Can you work these out from the model? Positions are in its coordinate system, mm. Give positions to 0.01 mm unless a question says otherwise; leave off trailing zeros. Write each loop counter-clockwise with the first axis right and the second up, starting at its lowest first coordinate (ties: lowest second). Pieces come first, ordered by that corner, then holes.
1. If I drill on probe 1 along Z at (x, y) = (89, 5); probe 2 along Z at (x, y) = (81.5, 1.5); probe 3 along X at (y, z) = (4.5, -451), over which ranges is the centre line in solid material (lowest first)?
2. Suppose I cut it at C-C (y = 4.5). Please give me the cut outline in (x, z).
3. I'm going to push flat-ended pins straight in: pin 1 (3 mm diameter, centred on x = 6.5, y = 4.5, fed in from -Z); pin 2 (3 mm diameter, centred on y = 4.5, z = -5, fed in from +X); pin 3 (2 mm diameter, centred on y = 1, z = -626, fed in from -X); pin 4 (3 mm diameter, centred on y = 4, z = -5, fed in from -X). Where does each tip first touch, or does it pass through?
4. Suppose I cut it at B-B (x = 66). Please give me the cut outline in (y, z).
5. Suppose I cut it at A-A (z = -383). Please give me the cut outline in (x, y), and give its area (3 significant figures).
```python
from build123d import *

# Parameters (mm, degrees)
SKETCH1_W           = 219.202
SKETCH1_H           = 879.7036
BOSS_EXTRUDE1_DEPTH = 6.35
SKETCH4_R           = 76.2
SKETCH4_W           = 8.89
SKETCH4_H           = 8.89
CUT_EXTRUDE3_DEPTH  = 907.624653954
FILLET1_R           = 0.254


with BuildPart() as part:
    # Sketch1 → Boss-Extrude1 (new body)
    with BuildSketch(Plane(origin=(0, 0, 0), x_dir=(1, 0, 0), z_dir=(0, 1, 0))):
        with Locations((109.601, 439.8518)):
            Rectangle(SKETCH1_W, SKETCH1_H)
    extrude(amount=BOSS_EXTRUDE1_DEPTH)

    # Sketch4 → Cut-Extrude3 (cut, through all)
    with BuildSketch(Plane(origin=(0, 6.35, 0), x_dir=(1, 0, 0), z_dir=(0, 1, 0))):
        with Locations(Location((86.6394, 439.8518, 0), (0, 0, 270))):
            Circle(SKETCH4_R)
        with Locations((4.445, 4.445)):
            Rectangle(SKETCH4_W, SKETCH4_H)
        with Locations((214.757, 4.445)):
            Rectangle(SKETCH4_W, SKETCH4_H)
        with Locations((214.757, 875.2586)):
            Rectangle(SKETCH4_W, SKETCH4_H)
        with Locations((4.445, 875.2586)):
            Rectangle(SKETCH4_W, SKETCH4_H)
    extrude(amount=-CUT_EXTRUDE3_DEPTH, mode=Mode.SUBTRACT)

    # Fillet1
    fillet1_edges = [part.edges().sort_by_distance(p)[0] for p in [
        (0, 3.175, -870.8136),
        (8.89, 3.175, -879.7036),
        (8.89, 3.175, -870.8136),
        (219.202, 3.175, -870.8136),
        (210.312, 3.175, -870.8136),
        (210.312, 3.175, -879.7036),
        (219.202, 3.175, -8.89),
        (210.312, 3.175, 0),
        (210.312, 3.175, -8.89),
        (0, 3.175, -8.89),
        (8.89, 3.175, -8.89),
        (8.89, 3.175, 0),
    ]]
    fillet(fillet1_edges, radius=FILLET1_R)


solid = part.part
```
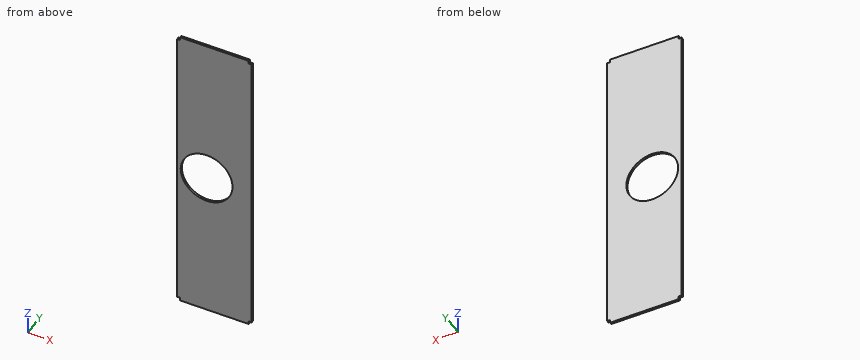
Checks:
1. probe 1: z = -879.7 to -516.02, -363.69 to 0
1. probe 2: z = -879.7 to -515.88, -363.83 to 0
1. probe 3: x = 0 to 11.26, 162.02 to 219.2
2. outline: (0, -870.56) arc R0.25 ccw to (0.25, -870.81) - (8.64, -870.81) arc R0.25 cw to (8.89, -871.07) - (8.89, -879.45) arc R0.25 ccw to (9.14, -879.7) - (210.06, -879.7) arc R0.25 ccw to (210.31, -879.45) - (210.31, -871.07) arc R0.25 cw to (210.57, -870.81) - (218.95, -870.81) arc R0.25 ccw to (219.2, -870.56) - (219.2, -9.14) arc R0.25 ccw to (218.95, -8.89) - (210.57, -8.89) arc R0.25 cw to (210.31, -8.64) - (210.31, -0.25) arc R0.25 ccw to (210.06, 0) - (9.14, 0) arc R0.25 ccw to (8.89, -0.25) - (8.89, -8.64) arc R0.25 cw to (8.64, -8.89) - (0.25, -8.89) arc R0.25 ccw to (0, -9.14) - close; hole circle Ø152.4 at (86.64, -439.85)
3. pin 1: stops at z = -870.81
3. pin 2: stops at x = 210.31
3. pin 3: stops at x = 0
3. pin 4: stops at x = 8.89
4. outline: (0, -879.7) - (6.35, -879.7) - (6.35, -513.2) - (0, -513.2) - close; (0, -366.5) - (6.35, -366.5) - (6.35, 0) - (0, 0) - close
5. outline: (0, 0) - (35.9, 0) - (35.9, 6.35) - (0, 6.35) - close; (137.38, 0) - (219.2, 0) - (219.2, 6.35) - (137.38, 6.35) - close
5. area: 748 mm2
